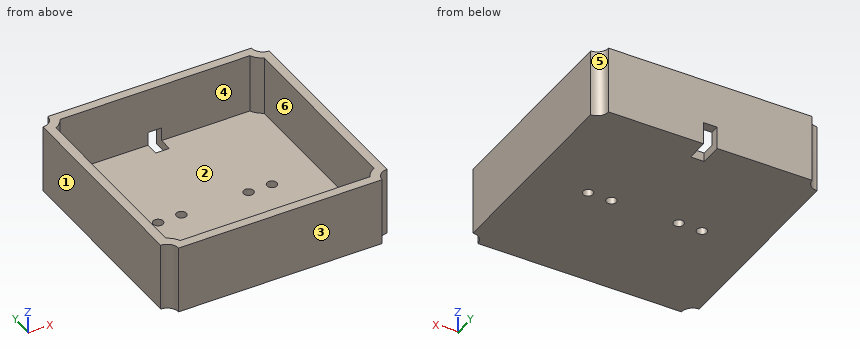
```python
from build123d import *

# Parameters (mm, degrees)
F0_R     = 1.1
F1_DEPTH = 5
F2_DEPTH = 10
F3_T     = -2
F4_W     = 3
F4_H     = 10
F5_DEPTH = 5


with BuildPart() as f1:
    # F0 (on Top) → F1 (new body)
    with BuildSketch(Plane.XY):
        with BuildLine():
            Line((-22.5, -25), (22.5, -25))
            ThreePointArc((22.5, -25), (23.232233047, -23.232233047), (25, -22.5))
            Line((25, -22.5), (25, 22.5))
            ThreePointArc((25, 22.5), (23.232233047, 23.232233047), (22.5, 25))
            Line((22.5, 25), (-22.5, 25))
            ThreePointArc((-22.5, 25), (-23.232233047, 23.232233047), (-25, 22.5))
            Line((-25, 22.5), (-25, -22.5))
            ThreePointArc((-25, -22.5), (-23.232233047, -23.232233047), (-22.5, -25))
        make_face()
        with BuildLine():
            ThreePointArc((-12.345503876, -1.0747146448), (-13.4367221651, 0.6899471949), (-11.48, 0))
            ThreePointArc((-11.48, 0), (-11.7232778349, -0.6899471949), (-12.345503876, -1.0747146448))
        make_face(mode=Mode.SUBTRACT)
        with Locations((-7.42, 0)):
            Circle(F0_R, mode=Mode.SUBTRACT)
        with Locations((7.42, 0)):
            Circle(F0_R, mode=Mode.SUBTRACT)
        with Locations((12.58, 0)):
            Circle(F0_R, mode=Mode.SUBTRACT)
    extrude(amount=F1_DEPTH)

    # F2 (add): a face of the model
    f2_faces = [f1.faces().sort_by_distance(p)[0] for p in [
        (0, 0, 5),
    ]]
    extrude(f2_faces, amount=F2_DEPTH)

    # F3
    f3_openings = [f1.faces().sort_by_distance(p)[0] for p in [
        (-13.68, 0, 2.5),
        (-13.68, 0, 10),
        (0, 0, 15),
        (11.48, 0, 2.5),
        (11.48, 0, 10),
        (6.32, 0, 2.5),
        (6.32, 0, 10),
        (-8.52, 0, 2.5),
        (-8.52, 0, 10),
    ]]
    offset(amount=F3_T, openings=f3_openings)

    # F4 (on Top) → F5 (cut)
    with BuildSketch(Plane.XY):
        with Locations((0, 25.013813749)):
            Rectangle(F4_W, F4_H)
    extrude(amount=F5_DEPTH, mode=Mode.SUBTRACT)


solid = f1.part
```
Check sheet for the modelled part. Datum: model origin and axes. Units: mm. Face numbers are marked on the shaded views. A direction names the side the tool comes from. Round coordinates to 2 decimals unless told otherwise and drop trailing zeros. Write each loop counter-clockwise with the first axis right and the second up, starting at its lowest first coordinate (ties: lowest second). Pieces come first, ordered by that corner, then holes. Notation, with made-up numbers: M 75.5,-19 L 131.5,-19 A17 cw 131.5,-11 Z; hole C -18,-25 d6. An arc over 180 degrees is marked long. Write item = value, one per line. Start each with the question number.
1. Section check B-B, the plane x = 12.58. Record the cut outline in (y, z), then the cut area to 3 significant figures.
2. Tool access check on the marked faces 5 and 6. Record the directions out of +Z, -Z, +X, -X, +Y, -Y that give a thin tool (end or side, any length) a straight path to the whole face; none if there is none.
3. Gauge pin test, flat ends, axial feed: pin 1 (1.5 mm diameter, centred on x = -16.5, y = 9.5, fed in from -Z); pin 2 (1.5 mm diameter, centred on y = 23.5, z = 1.5, fed in from -X); pin 3 (2.5 mm diameter, centred on x = -12.58, y = 0, fed in from +Z); pin 4 (0.6 mm diameter, centred on x = 0, y = 23.5, fed in from -Z). Record the tip position at first contact, or that the pin passes through.
4. Section check D-D, the plane y = 10. Record the cut outline in (x, z).
5. Section check A-A, the plane y = 0. Record the cut outline in (x, z), then the cut area to 3 significant figures.
6. Section check C-C, the plane z = 8. Record the cut outline in (x, y), then the cut area to 3 significant figures.
7. Release check for a two-part mould opening along X. For the marked faces 1, 2, 3 and 4 record: pulls with the +X half, pulls with the -X half, needs draft (parallel to the pull), parting line crosses it, or undercut.
8. Scan lines: line 1 (Y direction, x = -16.5, z = 6.5); line 2 (Y direction, x = -7.42, z = 1.05). Record each from-to range of solid material in increasing order. Write a range as [from, to].
Results found:
q1.outline = M -25,0 L -1.1,0 L -1.1,2 L -23,2 L -23,15 L -25,15 Z; M 1.1,0 L 25,0 L 25,15 L 23,15 L 23,2 L 1.1,2 Z
q1.area = 148 mm^2
q2.face_5 = +Z, -Z, +X, +Y
q2.face_6 = +Z
q3.pin_1 = 0
q3.pin_2 = -23.91
q3.pin_3 = 2
q3.pin_4 = 5
q4.outline = M -25,0 L 25,0 L 25,15 L 23,15 L 23,2 L -23,2 L -23,15 L -25,15 Z
q5.outline = M -25,0 L -13.68,0 L -13.68,2 L -23,2 L -23,15 L -25,15 Z; M -11.48,0 L -8.52,0 L -8.52,2 L -11.48,2 Z; M -6.32,0 L 6.32,0 L 6.32,2 L -6.32,2 Z; M 8.52,0 L 11.48,0 L 11.48,2 L 8.52,2 Z; M 13.68,0 L 25,0 L 25,15 L 23,15 L 23,2 L 13.68,2 Z
q5.area = 134 mm^2
q6.outline = M -25,-22.5 A2.5 cw -22.5,-25 L 22.5,-25 A2.5 cw 25,-22.5 L 25,22.5 A2.5 cw 22.5,25 L -22.5,25 A2.5 cw -25,22.5 Z; hole M -23,-20.97 A4.5 cw -20.97,-23 L 20.97,-23 A4.5 cw 23,-20.97 L 23,20.97 A4.5 cw 20.97,23 L -20.97,23 A4.5 cw -23,20.97 Z
q6.area = 374 mm^2
q7.face_1 = pulls with the -X half
q7.face_2 = undercut
q7.face_3 = needs draft
q7.face_4 = undercut
q8.line_1 = [-25, -23], [23, 25]
q8.line_2 = [-25, -1.1], [1.1, 25]
